Verification items for this drawing (mm, ordinates from the low corner). Give positions to 0.01 mm unless a question says otherwise; leave off trailing zeros. Loops run counter-clockwise (first coordinate to the right, second up) from the corner with the lowest first, then second, coordinate; pieces in that order, holes last. Notation, with made-up numbers: (-27, 38) - (21, 38) arc R30 ccw to (21, 71) - close; hole circle Ø11 at (-14, -32). An arc over 180 degrees is marked (long way). Write item = value, one per line. Start each with the question number.
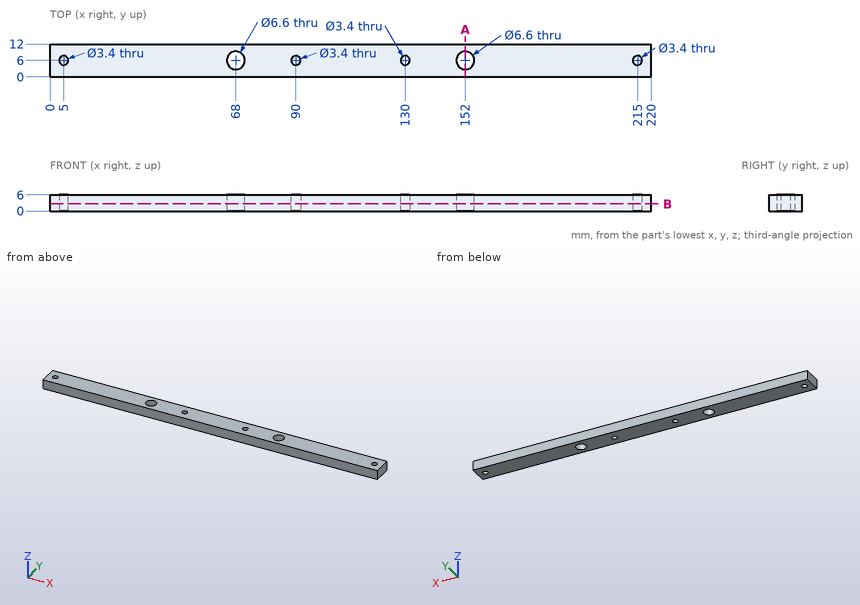
1) Cross-section at B-B on z = 2.65. Enter the section's corners in (x, y), and give its area (3 significant figures).
2) Material ranges on line 1 along Y through (x, z) = (130, 1.8); line 2 along X through (y, z) = (8.25, 5.15); line 3 along X through (y, z) = (8.5, 5.75), recorded low to high.
3) Cross-section at A-A on x = 152. Enter the section's corners in (y, z).
Checked values:
q1.outline = (0, 0) - (220, 0) - (220, 12) - (0, 12) - close; hole circle Ø3.4 at (5, 6); hole circle Ø6.6 at (68, 6); hole circle Ø3.4 at (90, 6); hole circle Ø3.4 at (130, 6); hole circle Ø6.6 at (152, 6); hole circle Ø3.4 at (215, 6)
q1.area = 2,540 mm²
q2.line_1 = 0 to 4.3, 7.7 to 12
q2.line_2 = 0 to 65.59, 70.41 to 149.59, 154.41 to 220
q2.line_3 = 0 to 65.85, 70.15 to 149.85, 154.15 to 220
q3.outline = (0, 0) - (2.7, 0) - (2.7, 6) - (0, 6) - close; (9.3, 0) - (12, 0) - (12, 6) - (9.3, 6) - close
